```python
from build123d import *

# Parameters (mm, degrees)
SKETCH2_R          = 19.05
SKETCH2_R_2        = 6.35
CUT_EXTRUDE1_DEPTH = 113.567071735


with BuildPart() as part:
    # Sketch1 → Revolve1 (revolve)
    with BuildSketch(Plane(origin=(0, 0, 0), x_dir=(0, 0, -1), z_dir=(1, 0, 0))):
        with BuildLine():
            Line((34.925, 28.575), (34.925, 6.35))
            ThreePointArc((34.925, 6.35), (33.065128061, 1.859871939), (28.575, 0))
            Line((28.575, 0), (0, 0))
            Line((0, 0), (0, 53.975))
            Line((0, 53.975), (69.85, 53.975))
            Line((69.85, 53.975), (69.85, 41.275))
            ThreePointArc((69.85, 41.275), (67.990128061, 36.784871939), (63.5, 34.925))
            Line((63.5, 34.925), (41.275, 34.925))
            ThreePointArc((41.275, 34.925), (36.784871939, 33.065128061), (34.925, 28.575))
        make_face()
    revolve(axis=Axis((0, 0, 0), (0, 1, 0)))

    # Sketch2 → Cut-Extrude1 (cut, through all)
    with BuildSketch(Plane(origin=(0, 53.975, 0), x_dir=(1, 0, 0), z_dir=(0, 1, 0))):
        with Locations(Location((0, 0, 0), (0, 0, 270))):
            Circle(SKETCH2_R)
        with Locations(Location((0, 53.975, 0), (0, 0, 270))):
            Circle(SKETCH2_R_2)
        with Locations(Location((53.975, 0, 0), (0, 0, 270))):
            Circle(SKETCH2_R_2)
        with Locations(Location((0, -53.975, 0), (0, 0, 270))):
            Circle(SKETCH2_R_2)
        with Locations(Location((-53.975, 0, 0), (0, 0, 270))):
            Circle(SKETCH2_R_2)
    extrude(amount=-CUT_EXTRUDE1_DEPTH, mode=Mode.SUBTRACT)


solid = part.part
```
Input: part model. Units: mm. Frame: model coordinates. A direction names the side the tool comes from. Round coordinates to 2 decimals unless told otherwise and drop trailing zeros. Loops run counter-clockwise (first coordinate to the right, second up) from the corner with the lowest first, then second, coordinate; pieces in that order, holes last. Notation, with made-up numbers: (28, 81.5) -> (55, 81.5) arc R21 ccw to (55, 91.5) -> close; hole circle Ø2 at (-13, -16.75). An arc over 180 degrees is marked (long way). Use one line per item in the form item = value. Start each with the question number.
Item 1: Material intervals for L1, parallel to X at y = 50, z = 0 (3 decimals); L2, parallel to X at y = 20.5, z = 0 (3 decimals); L3, parallel to Y at x = 28, z = 47 (3 decimals), sorted ascending. Write a range as from..to.
Item 2: Section query C-C on y = 20. Return the cut outline in (x, z) (3 decimals), then the cut area to 3 significant figures.
Item 3: Set-up query: faces 4 (the face through (19, 0, -6)), 5 (the face through (21.251, 17.307, 27.715)). Return all of +Z, -Z, +X, -X, +Y, -Y with unobstructed straight access to the full face (end or side cutting, diameter ignored); none if empty.
Item 4: Contact query for flat-ended pins moving along their axis: pin 1 Ø12 at (x, z) = (42.5, -14) entering from -Y; pin 2 Ø7.5 at (x, z) = (-53.975, 0) entering from -Y; pin 3 Ø6 at (x, z) = (-5.5, 49) entering from -Y (3 decimals); pin 4 Ø3 at (x, y) = (31, 46) entering from +Z. Output: stop coordinate, or through.
Item 5: Section query A-A on z = 0. Return the cut outline in (x, y) (3 decimals).
Item 6: Section query B-B on x = 0. Return the cut outline in (y, z) (3 decimals), then the cut area to 3 significant figures.
Item 7: Mould query, pull axis Z, two halves, no side actions, for faces 1 (the face through (-11.59, 27.37, -15.12)), 2 (the face through (-0.89, 34.925, -41.44)), 3 (the face through (42.503, 47.536, 55.431)). Classes: pulls with the +Z half, pulls with the -Z half, needs draft (parallel to the pull), parting line crosses it, or undercut.
Ans:
q1.L1 = -69.85..-60.325, -47.625..-19.05, 19.05..47.625, 60.325..69.85
q1.L2 = -34.925..-19.05, 19.05..34.925
q1.L3 = 34.925..53.975
q2.outline = circle Ø69.85 at (0, 0); hole circle Ø38.1 at (0, 0)
q2.area = 2,690 mm^2
q3.face_4 = +Z, -Z, +X, -X, -Y
q3.face_5 = -Y
q4.pin_1 = 34.4
q4.pin_2 = through
q4.pin_3 = 34.925
q4.pin_4 = 63.31
q5.outline = (-69.85, 41.275) arc R6.35 ccw to (-63.5, 34.925) -> (-60.325, 34.925) -> (-60.325, 53.975) -> (-69.85, 53.975) -> close; (-47.625, 34.925) -> (-41.275, 34.925) arc R6.35 cw to (-34.925, 28.575) -> (-34.925, 6.35) arc R6.35 ccw to (-28.575, 0) -> (-19.05, 0) -> (-19.05, 53.975) -> (-47.625, 53.975) -> close; (19.05, 0) -> (28.575, 0) arc R6.35 ccw to (34.925, 6.35) -> (34.925, 28.575) arc R6.35 cw to (41.275, 34.925) -> (47.625, 34.925) -> (47.625, 53.975) -> (19.05, 53.975) -> close; (60.325, 34.925) -> (63.5, 34.925) arc R6.35 ccw to (69.85, 41.275) -> (69.85, 53.975) -> (60.325, 53.975) -> close
q6.outline = (0, -28.575) arc R6.35 ccw to (6.35, -34.925) -> (28.575, -34.925) arc R6.35 cw to (34.925, -41.275) -> (34.925, -47.625) -> (53.975, -47.625) -> (53.975, -19.05) -> (0, -19.05) -> close; (0, 19.05) -> (53.975, 19.05) -> (53.975, 47.625) -> (34.925, 47.625) -> (34.925, 41.275) arc R6.35 cw to (28.575, 34.925) -> (6.35, 34.925) arc R6.35 ccw to (0, 28.575) -> close; (34.925, -63.5) arc R6.35 ccw to (41.275, -69.85) -> (53.975, -69.85) -> (53.975, -60.325) -> (34.925, -60.325) -> close; (34.925, 60.325) -> (53.975, 60.325) -> (53.975, 69.85) -> (41.275, 69.85) arc R6.35 ccw to (34.925, 63.5) -> close
q6.area = 2,540 mm^2
q7.face_1 = undercut
q7.face_2 = needs draft
q7.face_3 = parting line crosses it
